Design review of the part built by this model. Coordinates are the model's own, in mm. Coordinates: 2 decimals unless noted, no trailing zeros. Write each loop counter-clockwise with the first axis right and the second up, starting at its lowest first coordinate (ties: lowest second). Pieces come first, ordered by that corner, then holes. Notation, with made-up numbers: (73, 65) - (130, 65) arc R3 ccw to (130, 70) - close; hole circle Ø3 at (-36.75, -25.5). An arc over 180 degrees is marked (long way). Use a Markdown table: item, result.
Autodesk Inventor part; units mm, degrees
ref_plane "YZ Plane" through (0, 0, 0) normal (1, 0, 0) x (0, 1, 0)
ref_plane "XZ Plane" through (0, 0, 0) normal (0, 1, 0) x (-1, 0, 0)
ref_plane "XY Plane" through (0, 0, 0) normal (0, 0, 1) x (1, 0, 0)
sketch "Sketch1" plane through (0, 0, 0) normal (0, 1, 0) x (-1, 0, 0)
  line L0 (3.175, 0) -> (3.175, 165.1)
  line L1 (3.175, 165.1) -> (0, 165.1)
  line L2 (0, 165.1) -> (0, 190.5)
  line L3 (0, 190.5) -> (-8.89, 190.5)
  line L4 (-8.89, 190.5) -> (-8.89, 165.1)
  line L5 (-8.89, 165.1) -> (-12.065, 165.1)
  line L6 (-12.065, 165.1) -> (-12.065, -165.1)
  line L7 (-12.065, -165.1) -> (-8.89, -165.1)
  line L8 (-8.89, -165.1) -> (-8.89, -190.5)
  line L9 (-8.89, -190.5) -> (0, -190.5)
  line L10 (0, -190.5) -> (0, -165.1)
  line L11 (0, -165.1) -> (3.175, -165.1)
  line L12 (3.175, -165.1) -> (3.175, 0)
  point P0 (0, 0)
  dimension "d0" = 165.1
  dimension "d1" = 3.175
  dimension "d2" = 25.4
  dimension "d3" = 8.89
  dimension "d4" = 25.4
  dimension "d5" = 3.175
  dimension "d6" = 90
  dimension "d7" = 330.2
  dimension "d8" = 3.175
  dimension "d9" = 25.4
  dimension "d10" = 8.89
  dimension "d11" = 25.4
  dimension "d12" = 3.175
extrude "Extrusion1" add sketch "Sketch1" along normal blind 3.175
properties part number "front"
(1) For L1, parallel to Z at x = -0.5, y = 1.3; L2, parallel to X at y = 0.7, z = -166.5, list the stretches that pass through material, from the lowest coordinate up. Write a range as from..to.
Determined:
| item | result |
|---|---|
| L1 | -165.1..165.1 |
| L2 | 0..8.89 |
(2) Take a section at A-A on y = 2.05. Write out the cut boundary in (x, z) (3 decimals).
Determined:
| item | result |
|---|---|
| outline | (-3.175, -165.1) - (0, -165.1) - (0, -190.5) - (8.89, -190.5) - (8.89, -165.1) - (12.065, -165.1) - (12.065, 165.1) - (8.89, 165.1) - (8.89, 190.5) - (0, 190.5) - (0, 165.1) - (-3.175, 165.1) - close |
(3) For pin 1 (1.6 mm diameter, centred on y = 1, z = -180, fed in from -X); pin 2 (1 mm diameter, centred on x = 10, y = 1, fed in from -Z); pin 3 (1.6 mm diameter, centred on y = 1, z = 178.5, fed in from +X), all flat-tipped, find the tip position at first contact; note any pin that passes through.
Determined:
| item | result |
|---|---|
| pin 1 | x = 0 |
| pin 2 | z = -165.1 |
| pin 3 | x = 8.89 |
